Design review of the part shown in the three views and the two pictorial views. Dimensions are in mm from the part's minimum x, y and z. Coordinates: 2 decimals unless noted, no trailing zeros. Loops run counter-clockwise (first coordinate to the right, second up) from the corner with the lowest first, then second, coordinate; pieces in that order, holes last. Notation, with made-up numbers: (16.25, 30) -> (55.25, 30) arc R28 ccw to (55.25, 65) -> close; hole circle Ø8 at (-3.5, 64.5). An arc over 180 degrees is marked (long way). One line per item, written item: value. Start each with the question number.
1. Add section D-D on x = 3.5. Write out the cut boundary in (y, z), plus the area to 3 significant figures.
2. Insertion check: pin 1 (3 mm diameter, centred on y = 10, z = 17, fed in from -X); pin 2 (1.5 mm diameter, centred on y = 9, z = 11.5, fed in from +X); pin 3 (0.8 mm diameter, centred on x = 15, y = 13, fed in from -Z) (1 decimal); pin 4 (8 mm diameter, centred on y = 4, z = 14, fed in from -X). Each pin has a flat end and moves straight along its axis. Give the tip position at first contact, or say it passes through.
3. Add section A-A on x = 12. Write out the cut boundary in (y, z) (1 decimal), plus the area to 3 significant figures.
4. Add section C-C on y = 7.5. Write out the cut boundary in (x, z).
5. For probe 1 along Y at (x, z) = (13.25, 11); probe 2 along X at (y, z) = (13.25, 16.5) (1 decimal); probe 3 along Z at (x, y) = (15.5, 5.75), list the stretches that pass through material, from the lowest coordinate up.
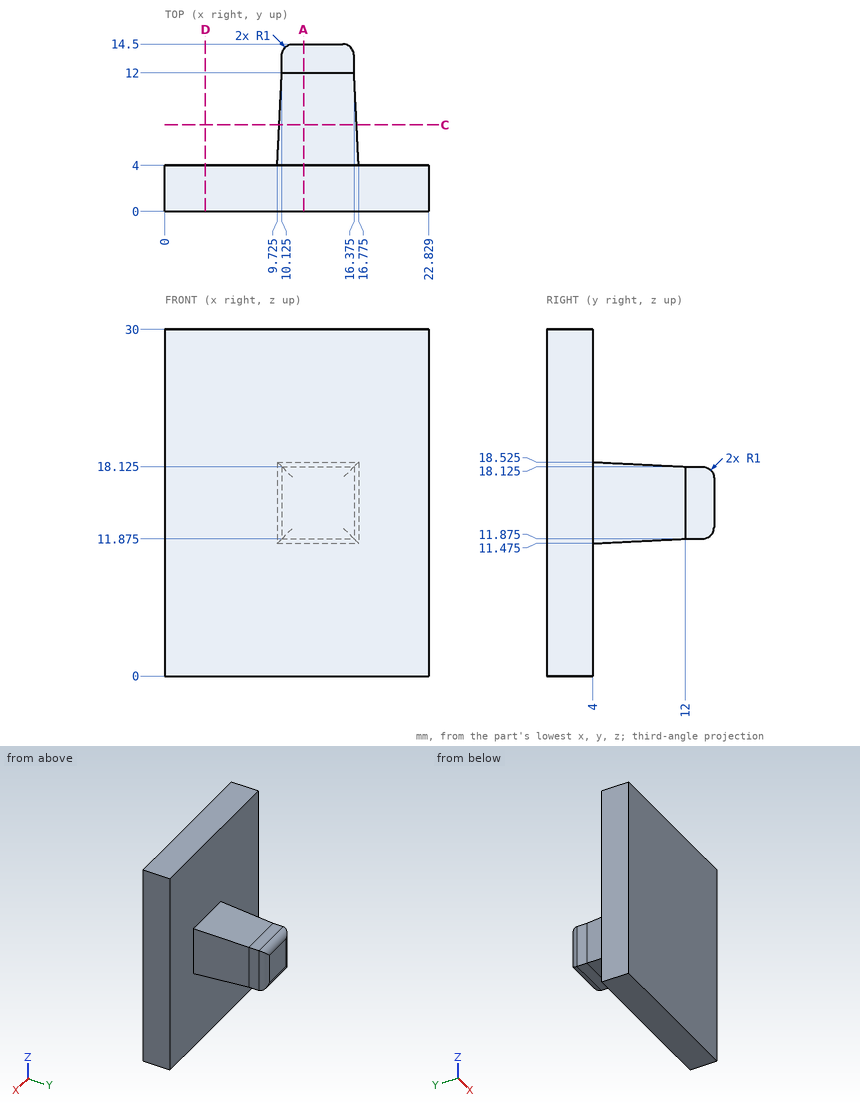
Worked answers:
1. outline: (0, 0) -> (4, 0) -> (4, 30) -> (0, 30) -> close
1. area: 120 mm²
2. pin 1: stops at x = 9.95
2. pin 2: stops at x = 16.56
2. pin 3: stops at z = 11.9
2. pin 4: stops at x = 0
3. outline: (0, 0) -> (4, 0) -> (4, 11.5) -> (12, 11.9) -> (13.5, 11.9) arc R1 ccw to (14.5, 12.9) -> (14.5, 17.1) arc R1 ccw to (13.5, 18.1) -> (12, 18.1) -> (4, 18.5) -> (4, 30) -> (0, 30) -> close
3. area: 188 mm²
4. outline: (9.9, 11.65) -> (16.6, 11.65) -> (16.6, 18.35) -> (9.9, 18.35) -> close
5. probe 1: y = 0 to 4
5. probe 2: x = 10.1 to 16.4
5. probe 3: z = 11.56 to 18.44
